Design review of the part built by this model. Coordinates are the model's own, in mm. Round coordinates to 2 decimals unless told otherwise and drop trailing zeros. Order: outer loops, then holes, each group sorted by start corner. A loop starts at its lowest first (then second) coordinate and runs counter-clockwise, first axis right, second up.
from build123d import *

# Parameters (mm, degrees)
SKETCH1_R           = 3.175
BOSS_EXTRUDE1_DEPTH = 25.4


with BuildPart() as part:
    # Sketch1 → Boss-Extrude1 (new body)
    with BuildSketch(Plane.XZ.offset(25.4)):
        with BuildLine():
            Line((-4.682174209, -4.59023638), (-3.666174209, -6.35))
            Line((-3.666174209, -6.35), (-1.634174209, -6.35))
            ThreePointArc((-1.634174209, -6.35), (0, -4.715825791), (1.634174209, -6.35))
            Line((1.634174209, -6.35), (3.666174209, -6.35))
            Line((3.666174209, -6.35), (4.682174209, -4.59023638))
            ThreePointArc((4.682174209, -4.59023638), (4.084024935, -2.357912895), (6.316348419, -1.75976362))
            Line((6.316348419, -1.75976362), (7.332348419, 0))
            Line((7.332348419, 0), (6.316348419, 1.75976362))
            ThreePointArc((6.316348419, 1.75976362), (4.084024935, 2.357912895), (4.682174209, 4.59023638))
            Line((4.682174209, 4.59023638), (3.666174209, 6.35))
            Line((3.666174209, 6.35), (1.634174209, 6.35))
            ThreePointArc((1.634174209, 6.35), (0, 4.715825791), (-1.634174209, 6.35))
            Line((-1.634174209, 6.35), (-3.666174209, 6.35))
            Line((-3.666174209, 6.35), (-4.682174209, 4.59023638))
            ThreePointArc((-4.682174209, 4.59023638), (-4.084024935, 2.357912895), (-6.316348419, 1.75976362))
            Line((-6.316348419, 1.75976362), (-7.332348419, 0))
            Line((-7.332348419, 0), (-6.316348419, -1.75976362))
            ThreePointArc((-6.316348419, -1.75976362), (-4.084024935, -2.357912895), (-4.682174209, -4.59023638))
        make_face()
        Circle(SKETCH1_R, mode=Mode.SUBTRACT)
    extrude(amount=-BOSS_EXTRUDE1_DEPTH)


solid = part.part
1) Take a section at B-B on x = 0. Give the boundary of the cut face in (y, z) (3 decimals), plus the area to 3 significant figures.
Results:
outline: (-25.4, -4.716) - (0, -4.716) - (0, -3.175) - (-25.4, -3.175) - close; (-25.4, 3.175) - (0, 3.175) - (0, 4.716) - (-25.4, 4.716) - close
area: 78.3 mm2
2) To check wall thickness, follow line 1 along Z through (x, y) = (0, -17) (3 decimals); line 2 along X through (y, z) = (-24.5, 6.25); line 3 along Z through (x, y) = (2.5, -2.5). State the ranges of each line that lie inside material, in increasing order.
Results:
line 1: z = -4.716 to -3.175, 3.175 to 4.716
line 2: x = -3.72 to -1.63, 1.63 to 3.72
line 3: z = -6.35 to -1.96, 1.96 to 6.35
3) Take a section at C-C on x = 4.25. Give the boundary of the cut face in (y, z).
Results:
outline: (-25.4, -5.34) - (0, -5.34) - (0, -4.23) - (-25.4, -4.23) - close; (-25.4, -2.12) - (0, -2.12) - (0, 2.12) - (-25.4, 2.12) - close; (-25.4, 4.23) - (0, 4.23) - (0, 5.34) - (-25.4, 5.34) - close
4) Take a section at A-A on y = -14.5. Give the boundary of the cut face in (x, z) (3 decimals), plus the area to 3 significant figures.
Results:
outline: (-7.332, 0) - (-6.316, -1.76) arc R1.634 cw to (-4.682, -4.59) - (-3.666, -6.35) - (-1.634, -6.35) arc R1.634 cw to (1.634, -6.35) - (3.666, -6.35) - (4.682, -4.59) arc R1.634 cw to (6.316, -1.76) - (7.332, 0) - (6.316, 1.76) arc R1.634 cw to (4.682, 4.59) - (3.666, 6.35) - (1.634, 6.35) arc R1.634 cw to (-1.634, 6.35) - (-3.666, 6.35) - (-4.682, 4.59) arc R1.634 cw to (-6.316, 1.76) - close; hole circle Ø6.35 at (0, 0)
area: 82.8 mm2
5) Take a section at D-D on z = -2.25. Give the boundary of the cut face in (x, y).
Results:
outline: (-4.15, -25.4) - (-2.24, -25.4) - (-2.24, 0) - (-4.15, 0) - close; (2.24, -25.4) - (4.15, -25.4) - (4.15, 0) - (2.24, 0) - close
6) Clearance check with flat-ended pins moving along their axes: P1, Ø4, axis at y = -3.5, z = -4, coming from the +X side; P2, Ø1, axis at x = -5.5, y = -9.5, coming from the +Z side; P3, Ø1, axis at x = -3, z = 4, coming from the +Y side. State where each tip first meets the part, or that it passes through.
Results:
P1: stops at x = 4.68
P2: stops at z = 1.62
P3: stops at y = 0
7) The part is to be moulded in two halves that separate along Z. For faces 1 (the face through (2, -25.4, 3)), 2 (the face through (-4.18, -12.88, -5.46)), 3 (the face through (-0.69, -12.88, -3.1)), say which applies: released by +Z, released by -Z, zero draft, split by the parting line, or undercut.
Results:
face 1: zero draft
face 2: released by -Z
face 3: undercut
